Geometry: final body of the model. Coordinates: model frame, mm. A direction names the side the tool comes from. Round coordinates to 2 decimals unless told otherwise and drop trailing zeros. Order: outer loops, then holes, each group sorted by start corner. A loop starts at its lowest first (then second) coordinate and runs counter-clockwise, first axis right, second up. Notation, with made-up numbers: M 28.5,51.5 L 50.5,51.5 A22 cw 50.5,71.5 Z; hole C 22,-25.75 d6. An arc over 180 degrees is marked long. Return JSON: item names as keys, results as strings. Group by question number.
Q1. Cut plane B-B on y = 17. Output: boundary loops of the cut face in (x, z), and give its area (3 significant figures).
Q2. Cut plane C-C on y = 14. Output: boundary loops of the cut face in (x, z), and give its area (3 significant figures).
Q3. Contact query for flat-ended pins moving along their axis: pin 1 (1.5 mm diameter, centred on y = 16, z = 4, fed in from -X); pin 2 (12 mm diameter, centred on y = 18.5, z = 6, fed in from +X); pin 3 (10 mm diameter, centred on y = 8.5, z = 4, fed in from -X); pin 4 (1 mm diameter, centred on x = 5.5, y = 16, fed in from -Z). Output: stop coordinate, or through.
Q4. Ray query, probe 1 along Z at (x, y) = (0, 5.25); probe 2 along X at (y, z) = (15.75, 0); probe 3 along Y at (x, z) = (6, 7.25). Return the intervals inside material, ascending.
Q5. Access query for faces 1 (the face through (5, 0, -2)), 2 (the face through (4, 15, -7)). Directions: +Z, -Z, +X, -X, +Y, -Y. A direction counts if a zero-diameter tool reaches every point of the face in a straight line with its end or side. Return the directions, or none.
Autodesk Inventor part; units mm, degrees
ref_plane "YZ Plane" through (0, 0, 0) normal (1, 0, 0) x (0, 1, 0)
ref_plane "XZ Plane" through (0, 0, 0) normal (0, 1, 0) x (-1, 0, 0)
ref_plane "XY Plane" through (0, 0, 0) normal (0, 0, 1) x (1, 0, 0)
sketch "Sketch1" plane through (0, 0, 0) normal (0, 1, 0) x (-1, 0, 0)
  circle A0 centre (0, 0) radius 7.5
  circle A1 centre (0, 0) radius 5.1
  dimension "d0" = 15
  dimension "d1" = 10.2
extrude "Extrusion1" add sketch "Sketch1" along normal blind 15
sketch "Sketch2" plane through (0, 15, 0) normal (0, 1, 0) x (1, 0, 0)
  circle A0 centre (0, 0) radius 7.5
  circle A1 centre (0, 0) radius 7.5
  circle A2 centre (0, 0) radius 5.1
  circle A3 centre (0, 0) radius 10
  dimension "d4" = 20
extrude "Extrusion2" add sketch "Sketch2" along normal blind 6 contours A0 | A3
chamfer "Chamfer1" distance 0.5 angle 45 3 edges at (-5.1, 21, 0) (-10, 21, 0) (7.5, 0, 0)
properties part number "Bøsning_beam_bund_3DPrint"
Result sheet:
{
 "1": {"outline": "C 0,0 d20; hole C 0,0 d10.2", "area": "232 mm²"},
 "2": {"outline": "C 0,0 d15; hole C 0,0 d10.2", "area": "95.0 mm²"},
 "3": {"pin 1": "stops at x = -9.46", "pin 2": "stops at x = 10", "pin 3": "stops at x = -7.5", "pin 4": "stops at z = -8.66"},
 "4": {"probe 1": "z = -7.5 to -5.1, 5.1 to 7.5", "probe 2": "x = -10 to -5.1, 5.1 to 10", "probe 3": "y = 15 to 21"},
 "5": {"face 1": "+Z, -Z, +X, -X, -Y", "face 2": "-Y"}
}
